Geometry check sheet. Reference: the model listing, model coordinates, mm. Face numbers are marked on the shaded views. A direction names the side the tool comes from. Give positions to 0.01 mm unless a question says otherwise; leave off trailing zeros. Loops run counter-clockwise (first coordinate to the right, second up) from the corner with the lowest first, then second, coordinate; pieces in that order, holes last. Notation, with made-up numbers: (19.5, 31.5) -> (35.5, 31.5) arc R24 cw to (35.5, 68.5) -> close; hole circle Ø7 at (57, 42). An arc over 180 degrees is marked (long way). One line per question, with ' | ' between items.
from build123d import *

# Parameters (mm, degrees)
F0_W     = 101.6
F0_H     = 76.2
F1_DEPTH = 38.1
F2_R     = 7.453167
F2_R_2   = 7.587908
F2_R_3   = 7.50333
F2_R_4   = 7.364953
F3_DEPTH = 38.101
F4_W     = 25.4
F4_H     = 50.8
F6_W     = 12.7
F6_H     = 12.7
F8_R     = 5.08
F9_SIZE  = 5.08


with BuildPart() as f1:
    # F0 (on Top) → F1 (new body)
    with BuildSketch(Plane.XY):
        Rectangle(F0_W, F0_H)
    extrude(amount=F1_DEPTH)

    # F2 (on Top) → F3 (cut, through all)
    with BuildSketch(Plane.XY):
        with Locations((-38.1, 25.4)):
            Circle(F2_R)
        with Locations((-38.1, -25.4)):
            Circle(F2_R_2)
        with Locations((38.1, 25.4)):
            Circle(F2_R_3)
        with Locations((38.1, -25.4)):
            Circle(F2_R_4)
    extrude(amount=F3_DEPTH, mode=Mode.SUBTRACT)

    # F4 (on Front) → F5 (revolve)
    with BuildSketch(Plane.XZ):
        with Locations((-12.7, 63.5)):
            Rectangle(F4_W, F4_H)
    revolve(axis=Axis((0, 0, 63.5), (0, 0, 1)))

    # F6 (on Front) → F7 (revolve, cut)
    with BuildSketch(Plane.XZ):
        with Locations((-24.13, 63.5)):
            Rectangle(F6_W, F6_H)
    revolve(axis=Axis((0, 0, 88.9), (0, 0, -1)), mode=Mode.SUBTRACT)

    # F8
    f8_edges = [f1.edges().sort_by_distance(p)[0] for p in [
        (25.4, 0, 88.9),
        (25.4, 0, 38.1),
    ]]
    fillet(f8_edges, radius=F8_R)

    # F9
    f9_edges = [f1.edges().sort_by_distance(p)[0] for p in [
        (0, -38.1, 38.1),
        (50.8, 0, 38.1),
        (0, 38.1, 38.1),
        (-50.8, 0, 38.1),
    ]]
    chamfer(f9_edges, length=F9_SIZE)


solid = f1.part
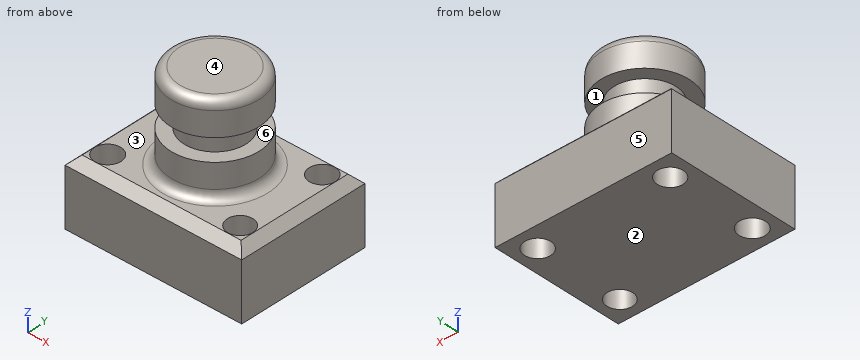
Item 1: Sectioned sample at C-C (z = 23.5). Record the cut outline in (x, y), plus the area to 3 significant figures.
Result:
outline: (-50.8, -38.1) -> (50.8, -38.1) -> (50.8, 38.1) -> (-50.8, 38.1) -> close; hole circle Ø15.18 at (-38.1, -25.4); hole circle Ø14.91 at (-38.1, 25.4); hole circle Ø15.01 at (38.1, 25.4); hole circle Ø14.73 at (38.1, -25.4) | area: 7,040 mm2
Item 2: Depth check by flat-ended pin: pin 1 Ø6 at (x, z) = (-8, 42) entering from +Y; pin 2 Ø5 at (x, z) = (5.5, 38.5) entering from -Y; pin 3 Ø3 at (y, z) = (2, 73.5) entering from -X; pin 4 Ø9 at (x, y) = (38.1, -25.4) entering from -Z. Enter the tip coordinate at first touch or a pass-through.
Result:
pin 1: y = 26.49 | pin 2: y = -35.12 | pin 3: x = -25.4 | pin 4: through
Item 3: Release check for a two-part mould opening along Z. For the marked faces 4, 5 and 6 record: pulls with the +Z half, pulls with the -Z half, needs draft (parallel to the pull), parting line crosses it, or undercut.
Result:
face 4: pulls with the +Z half | face 5: needs draft | face 6: undercut
Item 4: Sectioned sample at A-A (x = -38.1). Give the number of separate pieces and of enclosed holes in the cut face, plus the area to 3 significant figures.
Result:
separate pieces: 3 | enclosed holes: 0 | area: 1,730 mm2
Item 5: Sectioned sample at B-B (y = 0). Record the cut outline in (x, z), plus the area to 3 significant figures.
Result:
outline: (-50.8, 0) -> (50.8, 0) -> (50.8, 33.02) -> (45.72, 38.1) -> (30.48, 38.1) arc R5.08 cw to (25.4, 43.18) -> (25.4, 57.15) -> (17.78, 57.15) -> (17.78, 69.85) -> (25.4, 69.85) -> (25.4, 83.82) arc R5.08 ccw to (20.32, 88.9) -> (-20.32, 88.9) arc R5.08 ccw to (-25.4, 83.82) -> (-25.4, 69.85) -> (-17.78, 69.85) -> (-17.78, 57.15) -> (-25.4, 57.15) -> (-25.4, 43.18) arc R5.08 cw to (-30.48, 38.1) -> (-45.72, 38.1) -> (-50.8, 33.02) -> close | area: 6,230 mm2
Item 6: Scan lines: probe 1 along Y at (x, z) = (-38.1, 8.5); probe 2 along X at (y, z) = (-25, 9); probe 3 along Y at (x, z) = (38.1, 26). Record each from-to range of solid material in increasing order.
Result:
probe 1: -38.1 to -32.99, -17.81 to 17.95, 32.85 to 38.1 | probe 2: -50.8 to -45.68, -30.52 to 30.75, 45.45 to 50.8 | probe 3: -38.1 to -32.76, -18.04 to 17.9, 32.9 to 38.1
Item 7: Set-up check for the marked faces 1, 2 and 3: record each of +Z, -Z, +X, -X, +Y, -Y from which the full face is reachable in a straight line by a thin tool's end or side.
Result:
face 1: none | face 2: -Z, +X, -X, +Y, -Y | face 3: +Z
Item 8: Sectioned sample at D-D (x = 38.1). Record the cut outline in (y, z), plus the area to 3 significant figures.
Result:
outline: (-38.1, 0) -> (-32.76, 0) -> (-32.76, 38.1) -> (-33.02, 38.1) -> (-38.1, 33.02) -> close; (-18.04, 0) -> (17.9, 0) -> (17.9, 38.1) -> (-18.04, 38.1) -> close; (32.9, 0) -> (38.1, 0) -> (38.1, 33.02) -> (33.02, 38.1) -> (32.9, 38.1) -> close | area: 1,740 mm2
